Check sheet for the drawn part. Datum: minimum x, y, z corner. Units: mm. A direction names the side the tool comes from. Round coordinates to 2 decimals unless told otherwise and drop trailing zeros. Loops run counter-clockwise (first coordinate to the right, second up) from the corner with the lowest first, then second, coordinate; pieces in that order, holes last. Notation, with made-up numbers: (14.25, 26.5) - (37.25, 26.5) arc R19 ccw to (37.25, 48.5) - close; hole circle Ø3 at (-32.75, 85). An arc over 180 degrees is marked (long way). Use CSV: the item, a comma, the result in double quotes.
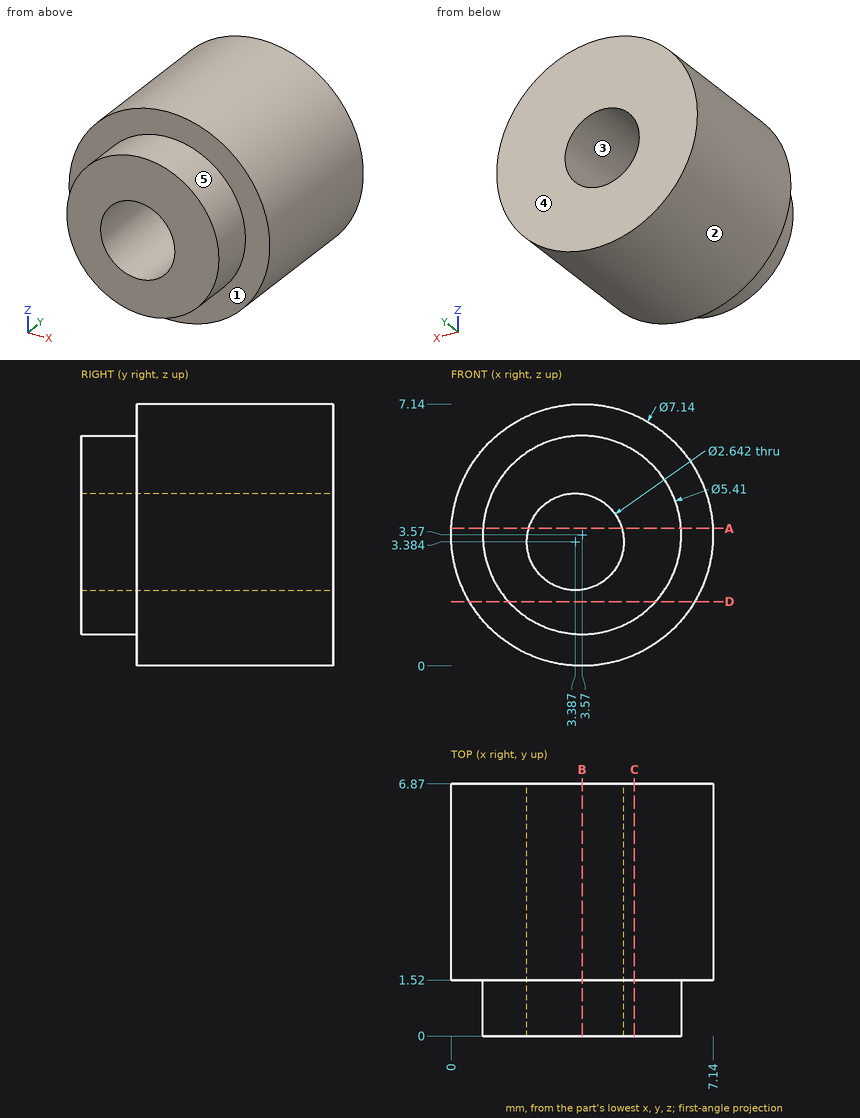
1) Cross-section at B-B, the plane x = 3.57. Record the cut outline in (y, z) (1 decimal).
Returned:
outline,"(0, 0.9) - (1.5, 0.9) - (1.5, 0) - (6.9, 0) - (6.9, 2.1) - (0, 2.1) - close; (0, 4.7) - (6.9, 4.7) - (6.9, 7.1) - (1.5, 7.1) - (1.5, 6.3) - (0, 6.3) - close"
2) Mould release check, pull along X, two halves, no side actions. Record for the marked faces 3, 4 and 5: +X half, -X half, draft (parallel to the pull), parting line (faces both ways), or undercut.
Returned:
face 3,"undercut"
face 4,"draft"
face 5,"parting line"
3) Access from +Z, -Z, +X, -X, +Y, -Y to the whole of each face (thin tool, end or side, straight path). Record for the marked faces 1 and 2.
Returned:
face 1,"-Y"
face 2,"+Y, -Y"
4) Thickness scan on probe 1 along Y at (x, z) = (6, 1.5); probe 2 along Z at (x, y) = (2.75, 6.5) (1 decimal); probe 3 along X at (y, z) = (4.5, 4.25) (1 decimal). Record the ranges inside material, lowest first. Write a range as [from, to].
Returned:
probe 1,"y = [1.52, 6.87]"
probe 2,"z = [0.1, 2.2], [4.5, 7]"
probe 3,"x = [0.1, 2.4], [4.4, 7.1]"
5) Cross-section at D-D, the plane z = 1.75. Record the cut outline in (x, y).
Returned:
outline,"(0.5, 1.52) - (1.57, 1.52) - (1.57, 0) - (5.57, 0) - (5.57, 1.52) - (6.64, 1.52) - (6.64, 6.87) - (0.5, 6.87) - close"
6) Cross-section at A-A, the plane z = 3.75. Record the cut outline in (x, y) (1 decimal), then the cut area to 3 significant figures.
Returned:
outline,"(0, 1.5) - (0.9, 1.5) - (0.9, 0) - (2.1, 0) - (2.1, 6.9) - (0, 6.9) - close; (4.7, 0) - (6.3, 0) - (6.3, 1.5) - (7.1, 1.5) - (7.1, 6.9) - (4.7, 6.9) - close"
area,"28.9 mm²"
7) Cross-section at C-C, the plane x = 5. Record the cut outline in (y, z), then the cut area to 3 significant figures.
Returned:
outline,"(0, 1.27) - (1.52, 1.27) - (1.52, 0.3) - (6.87, 0.3) - (6.87, 6.84) - (1.52, 6.84) - (1.52, 5.87) - (0, 5.87) - close"
area,"42.0 mm²"
8) Gauge pin test, flat ends, axial feed: pin 1 Ø1 at (x, y) = (1, 3.5) entering from +Z; pin 2 Ø1.5 at (x, y) = (2.5, 2) entering from +Z; pin 3 Ø2 at (x, y) = (3, 2.5) entering from -Z; pin 4 Ø1 at (y, z) = (3.5, 4.5) entering from -X. Record the tip position at first contact, or that the pin passes through.
Returned:
pin 1,"stops at z = 6.48"
pin 2,"stops at z = 7.13"
pin 3,"stops at z = 0"
pin 4,"stops at x = 0.03"
